Geometry: final body of the model. Coordinates: model frame, mm. Face numbers are marked on the shaded views. A direction names the side the tool comes from. Give positions to 0.01 mm unless a question says otherwise; leave off trailing zeros. Loops run counter-clockwise (first coordinate to the right, second up) from the corner with the lowest first, then second, coordinate; pieces in that order, holes last. Notation, with made-up numbers: (-3, 23) -> (34, 23) arc R10 cw to (34, 32) -> close; hole circle Ø5 at (24, -36.5). An arc over 180 degrees is marked (long way). One line per question, with ' | ' between items. Start each with the question number.
Item 1: Set-up query: the marked faces 5 and 6. Return all of +Z, -Z, +X, -X, +Y, -Y with unobstructed straight access to the full face (end or side cutting, diameter ignored); none if empty.
Item 2: Section A-A on x = 12. Return loops of the section in (y, z).
Item 3: Section B-B on z = -28. Return loops of the section in (x, y).
Item 4: Pin query (flat end, axial travel): P1, Ø5, axis at x = 18.5, y = 4.5, coming from the -Z side; P2, Ø4, axis at x = 27, y = -5, coming from the +Z side; P3, Ø5, axis at y = -3, z = 7.5, coming from the +X side. Return the tip coordinate at first contact, or that it passes through.
Item 5: Mould query, pull axis X, two halves, no side actions, for the marked faces 1, 2, 3 and 4. Classes: released by +X, released by -X, zero draft, split by the parting line, or undercut.
Item 6: Material intervals for line 1 along Z through (x, y) = (7, -9.5); line 2 along Y through (x, z) = (36, -22); line 3 along Z through (x, y) = (19.5, 9.75), sorted ascending. Write a range as [from, to].
Autodesk Inventor part; units mm, degrees
ref_plane "Work Plane2" through (23.3345, 0, 23.3345) normal (0.7071, 0, 0.7071) x (0, 1, 0)
ref_plane "XZ Plane" through (0, 0, 0) normal (0, 1, 0) x (-1, 0, 0)
ref_plane "XY Plane" through (0, 0, 0) normal (0, 0, 1) x (1, 0, 0)
sketch "Sketch1" plane through (0, 0, 0) normal (0, 0, 1) x (1, 0, 0)
  line L0 (0, 0) -> (0, 11.2) construction
  line L1 (0, 0) -> (20, 0) construction
  line L2 (20, 0) -> (20, 11) construction
  line L3 (0, 11.2) -> (0, 12.8)
  line L4 (0, 11.2) -> (20, 11)
  line L5 (0, 12.8) -> (20, 12.8)
  line L6 (0, 12.8) -> (20, 12.8) construction
  line L7 (20, 12.8) -> (20, 11)
  line L8 (20, 0) -> (25, 0) construction
  line L9 (25, 0) -> (25, 11.2) construction
  line L10 (25, 11.2) -> (20, 12.8)
  line L11 (25, 11.2) -> (25, 9.4)
  line L12 (25, 9.4) -> (20, 11)
  dimension "d0" = 11.2
  dimension "d1" = 20
  dimension "d2" = 11
  dimension "d3" = 1.6
  dimension "d4" = 0
  dimension "d5" = 5
  dimension "d6" = 11.2
  dimension "d7" = 1.8
revolve "Revolution1" add sketch "Sketch1" angle 360 about axis through (0, 0, 0) along (1, 0, 0)
sketch "Sketch2" plane through (25, 0, 0) normal (1, 0, 0) x (0, 0, -1)
  line L0 (0, 0) -> (11.2, 0) construction
  circle A0 centre (0, 0) radius 9.4
  circle A1 centre (0, 0) radius 11.2
  line L1 (11.2, 0) -> (11.2, 12.8) construction
  dimension "d9" = 11.2
revolve "Revolution2" add sketch "Sketch2" angle 90 about axis through (25, 0, -11.2) along (0, 1, 0)
sketch "Sketch3" plane through (0, 0, 0) normal (0, 1, 0) x (-1, 0, 0)
  line L0 (-47.4, -11.2) -> (-25, -11.2) construction
  line L1 (-36.2, -11.2) -> (-36.2, -31.2) construction
  line L2 (-36.2, -31.2) -> (-25.2, -31.2) construction
  line L3 (-25.2, -31.2) -> (-25, -11.2)
  line L4 (-25, -11.2) -> (-26.8, -11.2)
  arc A0 (-25, -9.4) -> (-26.8, -11.2) centre (-25, -11.2) ccw
  line L5 (-26.8, -11.2) -> (-26.8, -31.2)
  line L6 (-25.2, -31.2) -> (-26.8, -31.2)
  point P0 (0, 0)
  dimension "d11" = 20
  dimension "d12" = 11
revolve "Revolution3" add sketch "Sketch3" angle 360 about axis through (36.2, 0, -11.2) along (0, 0, -1)
ref_plane "Work Plane2" through (23.3345, 0, 23.3345) normal (0.7071, 0, 0.7071) x (0, 1, 0)
ref_plane "Work Plane1" through (0, 0, 0) normal (0.7071, 0, 0.7071) x (0, 1, 0)
sketch "Sketch4" plane through (23.3345, 0, 23.3345) normal (0.7071, 0, 0.7071) x (0, 1, 0)
  ellipse E0 centre (0, -17.6777) end of major axis (11.2, -17.6777) minor radius 7.9196 construction
  ellipse E1 centre (0, -33.5169) end of major axis (11.2, -33.5169) minor radius 7.9196 construction
  line L0 (0, -17.6777) -> (0, -33.5169) construction
  circle A0 centre (0, -25.5973) radius 10
  point P0 (0, 0)
  dimension "d16" = 20
extrude "Extrusion1" add sketch "Sketch4" against normal up to surface
equation "\"d0\" = 0.5 * TMEnd"
equation "\"d1\" = TDepth"
equation "\"d2\" = 0.5 * TMStart"
equation "\"d3\" = WallT"
equation "\"d6\" = 0.5 * TMEnd"
equation "\"d7\" = WallT + 0.5 * TMEnd - 0.5 * TMStart"
equation "\"d9\" = BendR"
equation "\"d11\" = TDepth"
equation "\"d12\" = 0.5 * TMStart"
properties part number "MtoF90Degree"
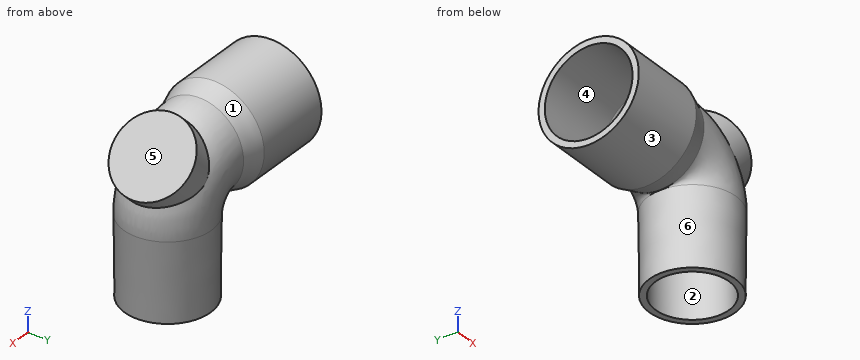
Result sheet:
1) face 5: +Z, +X, +Y, -Y | face 6: -Z
2) outline: circle Ø25.6 at (0, 0); hole circle Ø22.16 at (0, 0)
3) outline: circle Ø22.06 at (36.2, 0); hole circle Ø18.8 at (36.2, 0)
4) P1: stops at z = -12.64 | P2: stops at z = 10.72 | P3: stops at x = 41.67
5) face 1: undercut | face 2: undercut | face 3: zero draft | face 4: released by -X
6) line 1: z = [-8.58, -5.8], [5.8, 8.58] | line 2: y = [-11.09, -9.4], [9.4, 11.09] | line 3: z = [-8.29, -5.1], [5.1, 8.29]
